```python
from build123d import *

# Parameters (mm, degrees)
SCHIZZO1_W                   = 60
SCHIZZO1_H                   = 62
ESTRUSIONE_ESTRUSIONE1_DEPTH = 34
FORO_PER_VITE_M24_1_D        = 28
FORO1_D                      = 4.917
FORO1_DEPTH                  = 14.312635171
FORO1_TIP                    = 1.419415637
FORO2_D                      = 4.917
FORO2_DEPTH                  = 12.312635171
FORO2_TIP                    = 1.419415637
SMUSSO1_SIZE                 = 0.5415
SMUSSO2_SIZE                 = 2


with BuildPart() as part:
    # Schizzo1 → Estrusione-Estrusione1 (new body)
    with BuildSketch(Plane(origin=(17, 0, 0), x_dir=(0, 0, -1), z_dir=(1, 0, 0))):
        with Locations((0, 4)):
            Rectangle(SCHIZZO1_W, SCHIZZO1_H)
    extrude(amount=-ESTRUSIONE_ESTRUSIONE1_DEPTH)

    # Foro per Vite M24-1 (through all)
    with Locations(Plane(origin=(17, 0, 0), x_dir=(0, 0, -1), z_dir=(1, 0, 0))):
        with Locations((0, 0)):
            Hole(FORO_PER_VITE_M24_1_D / 2)

    # Foro1
    with Locations(Plane(origin=(0, 35, 0), x_dir=(1, 0, 0), z_dir=(0, 1, 0))):
        with Locations((9, 22.5), (9, -22.5), (-9, 22.5), (-9, -22.5)):
            Hole(FORO1_D / 2, depth=FORO1_DEPTH)
            with Locations((0, 0, -(FORO1_DEPTH + FORO1_TIP / 2))):  # 120° drill point
                Cone(0, FORO1_D / 2, FORO1_TIP, mode=Mode.SUBTRACT)

    # Foro2
    with Locations(Plane(origin=(17, 0, 0), x_dir=(0, 0, -1), z_dir=(1, 0, 0))):
        with Locations((13.435028843, 13.435028843), (-13.435028843, -13.435028843), (13.435028843, -13.435028843), (-13.435028843, 13.435028843)):
            Hole(FORO2_D / 2, depth=FORO2_DEPTH)
            with Locations((0, 0, -(FORO2_DEPTH + FORO2_TIP / 2))):  # 120° drill point
                Cone(0, FORO2_D / 2, FORO2_TIP, mode=Mode.SUBTRACT)

    # Smusso1
    smusso1_edges = [part.edges().sort_by_distance(p)[0] for p in [
        (-6.5415, 35, 22.5),
        (-6.5415, 35, -22.5),
        (11.4585, 35, 22.5),
        (11.4585, 35, -22.5),
        (17, 13.435028843, 10.976528843),
        (17, -13.435028843, -15.893528843),
        (17, -13.435028843, 10.976528843),
        (17, 13.435028843, -15.893528843),
    ]]
    chamfer(smusso1_edges, length=SMUSSO1_SIZE)

    # Smusso2
    smusso2_edges = [part.edges().sort_by_distance(p)[0] for p in [
        (0, -27, 30),
        (0, -27, -30),
    ]]
    chamfer(smusso2_edges, length=SMUSSO2_SIZE)


solid = part.part
```
Part model, mm, in its own coordinate system. A direction names the side the tool comes from. Round coordinates to 2 decimals unless told otherwise and drop trailing zeros. Loops run counter-clockwise (first coordinate to the right, second up) from the corner with the lowest first, then second, coordinate; pieces in that order, holes last. Notation, with made-up numbers: (52, 18.5) -> (93, 18.5) arc R19 ccw to (93, 34.5) -> close; hole circle Ø8 at (-26, 6). An arc over 180 degrees is marked (long way). Use a Markdown table: item, result.
1) Tool access for faces 1 (the cylindrical face through (10.491, -14.377, -11.164)), 2 (the cylindrical face through (-0.238, -5.362, 12.932)), 3 (the cylindrical face through (10.812, 27.477, 20.838)): list every direction of +Z, -Z, +X, -X, +Y, -Y with a clear straight run to the whole face (end or side of a thin tool).
The answers:
| item | result |
|---|---|
| face 1 | +X |
| face 2 | +X, -X |
| face 3 | +Y |
2) Cut at C-C, the plane z = 0. List the corners of the cut face in (x, y).
The answers:
| item | result |
|---|---|
| outline | (-17, -27) -> (17, -27) -> (17, -14) -> (-17, -14) -> close; (-17, 14) -> (17, 14) -> (17, 35) -> (-17, 35) -> close |
3) Probe line 1 (X direction, y = 29, z = -22.5); line 2 (Z direction, x = 9, y = 26); line 3 (Z direction, x = -7, y = 22). List the from-to ranges inside material, lowest first. Write a range as [from, to].
The answers:
| item | result |
|---|---|
| line 1 | x = [-17, -11.46], [-6.54, 6.54], [11.46, 17] |
| line 2 | z = [-30, -24.96], [-20.04, 20.04], [24.96, 30] |
| line 3 | z = [-30, -23.93], [-21.07, 21.07], [23.93, 30] |
4) Cut at A-A, the plane x = -1.5. List the corners of the cut face in (y, z), and give its area (3 significant figures).
The answers:
| item | result |
|---|---|
| outline | (-27, -28) -> (-25, -30) -> (35, -30) -> (35, 30) -> (-25, 30) -> (-27, 28) -> close; hole circle Ø28 at (0, 0) |
| area | 3,100 mm2 |
5) Cut at D-D, the plane y = 28.5. List the corners of the cut face in (x, z), and give its area (3 significant figures).
The answers:
| item | result |
|---|---|
| outline | (-17, -30) -> (17, -30) -> (17, 30) -> (-17, 30) -> close; hole circle Ø4.92 at (-9, -22.5); hole circle Ø4.92 at (-9, 22.5); hole circle Ø4.92 at (9, -22.5); hole circle Ø4.92 at (9, 22.5) |
| area | 1,960 mm2 |
6) Pull direction X, two halves, no side cores. Call faces 4 (the flat face through (0, -26, -29)), 5 (the conical face through (8.685, 19.514, 22.211)): pulls with the +X half, pulls with the -X half, needs draft (parallel to the pull), parting line crosses it, or undercut.
The answers:
| item | result |
|---|---|
| face 4 | needs draft |
| face 5 | undercut |
7) Drop flat-ended pins along their axis: pin 1 Ø5.5 at (y, z) = (13.44, -13.44) entering from +X; pin 2 Ø6.5 at (y, z) = (-13.44, 13.44) entering from +X; pin 3 Ø4.5 at (x, z) = (-9, -22.5) entering from +Y; pin 4 Ø3 at (x, z) = (-9, 22.5) entering from +Y. Give the stop position or say it passes through.
The answers:
| item | result |
|---|---|
| pin 1 | stops at x = 16.76 |
| pin 2 | stops at x = 17 |
| pin 3 | stops at y = 20.57 |
| pin 4 | stops at y = 20.13 |
8) Cut at B-B, the plane y = 0. List the corners of the cut face in (x, z), and give its area (3 significant figures).
The answers:
| item | result |
|---|---|
| outline | (-17, -30) -> (17, -30) -> (17, -14) -> (-17, -14) -> close; (-17, 14) -> (17, 14) -> (17, 30) -> (-17, 30) -> close |
| area | 1,090 mm2 |
